Model file for the job. Use its own axes, mm. A direction names the side the tool comes from. Round coordinates to 2 decimals unless told otherwise and drop trailing zeros. Loops run counter-clockwise (first coordinate to the right, second up) from the corner with the lowest first, then second, coordinate; pieces in that order, holes last. Notation, with made-up numbers: (-40, -17) -> (-17, -17) arc R14 cw to (-17, -12) -> close; hole circle Ø7 at (56.5, -34). An arc over 180 degrees is marked (long way). Use a Markdown table: item, result. Add a question column.
```python
from build123d import *

# Parameters (mm, degrees)
SKETCH1_W               = 355.325
SKETCH1_H               = 30
SKETCH1_R               = 12.5
SKETCH1_R_2             = 1
SKETCH1_W_2             = 50
SKETCH1_H_2             = 5
BOSS_EXTRUDE3_DEPTH     = 13
FILLET3_R               = 5
SKETCH3_R               = 12.5
BOSS_EXTRUDE4_DEPTH     = 13
CUT_EXTRUDE1_REACH      = 359.536
SKETCH4_R               = 1.425
SKETCH5_W               = 63.83
SKETCH5_H               = 18
CUT_EXTRUDE3_DEPTH      = 358.535810269
FILLET4_R               = 5
SKETCH6_W               = 63.8325
SKETCH6_H               = 17
CUT_EXTRUDE4_DEPTH      = 5
SKETCH7_R               = 2.159563788
SKETCH7_R_2             = 1
SKETCH7_R_3             = 2.117135705
SKETCH7_R_4             = 1.916104153
SKETCH7_R_5             = 2.415941568
BOSS_EXTRUDE5_DEPTH     = 8
SKETCH8_R               = 12.5
BOSS_EXTRUDE6_DEPTH     = 13
CUT_EXTRUDE5_DEPTH      = 358.535810269
CUT_EXTRUDE5_DEPTH_BACK = 358.535810269
SKETCH10_R              = 12.5
SKETCH10_R_2            = 13
SKETCH13_W              = 13
SKETCH13_H              = 30
BOSS_EXTRUDE7_DEPTH     = 5
SKETCH14_W              = 13
SKETCH14_H              = 9.8
BOSS_EXTRUDE8_DEPTH     = 5
SKETCH15_R              = 1.6
CUT_EXTRUDE6_DEPTH      = 357.119173347
SKETCH17_W              = 5
SKETCH17_H              = 30
CUT_EXTRUDE7_DEPTH      = 357.826085965
BOSS_EXTRUDE9_DEPTH     = 18.5
SKETCH19_W              = 13
SKETCH19_H              = 10.7
BOSS_EXTRUDE10_DEPTH    = 1
CUT_EXTRUDE8_REACH      = 373.267
SKETCH20_W              = 18.5
SKETCH20_H              = 0.75
SKETCH20_W_2            = 18.502042188


with BuildPart() as part:
    # Sketch1 → Boss-Extrude3 (new body)
    # profile 1 of 3: a face of its own
    with BuildSketch(Plane.XY):
        with Locations((177.6625, 15)):
            Rectangle(SKETCH1_W, SKETCH1_H)
        with Locations(Location((334.55, 14.5, 0), (0, 0, 180))):
            Circle(SKETCH1_R, mode=Mode.SUBTRACT)
        with Locations(Location((20.775, 14.5, 0), (0, 0, 180))):
            Circle(SKETCH1_R, mode=Mode.SUBTRACT)
    # profile 2 of 3: a face of its own
    with BuildSketch(Plane.XY):
        Polygon((177.6625, 0), (50, 0), (50, -5), (50, -17), (177.6625, -17), align=None)
        with Locations(Location((60, -14.5, 0), (0, 0, 180))):
            Circle(SKETCH1_R_2, mode=Mode.SUBTRACT)
        with Locations(Location((68, -14.5, 0), (0, 0, 180))):
            Circle(SKETCH1_R_2, mode=Mode.SUBTRACT)
        with Locations(Location((60, -2.5, 0), (0, 0, 180))):
            Circle(SKETCH1_R_2, mode=Mode.SUBTRACT)
        with Locations(Location((68, -2.5, 0), (0, 0, 180))):
            Circle(SKETCH1_R_2, mode=Mode.SUBTRACT)
    # profile 3 of 3: a face of its own
    with BuildSketch(Plane.XY):
        with Locations((25, -2.5)):
            Rectangle(SKETCH1_W_2, SKETCH1_H_2)
    extrude(amount=BOSS_EXTRUDE3_DEPTH)

    # Fillet3
    fillet3_edges = [part.edges().sort_by_distance(p)[0] for p in [
        (0, -5, 6.5),
        (0, 30, 6.5),
        (355.325, 30, 6.5),
        (355.325, 0, 6.5),
        (177.6625, -17, 6.5),
        (50, -17, 6.5),
    ]]
    fillet(fillet3_edges, radius=FILLET3_R)

    # Sketch3 → Boss-Extrude4 (add)
    with BuildSketch(Plane.XY.offset(13)):
        with Locations(Location((85, 14.5, 0), (0, 0, 180))):
            Circle(SKETCH3_R)
        with Locations(Location((165, 14.5, 0), (0, 0, 180))):
            Circle(SKETCH3_R)
        with Locations(Location((245, 14.5, 0), (0, 0, 180))):
            Circle(SKETCH3_R)
    extrude(amount=BOSS_EXTRUDE4_DEPTH)

    # Sketch4 → Cut-Extrude1 (cut, up to next)
    with BuildSketch(Plane(origin=(0, 0, 0), x_dir=(-1, 0, 0), z_dir=(0, 0, -1)), mode=Mode.PRIVATE) as cut_extrude1_sk1:
        with Locations((-68, -2.5)):
            Circle(SKETCH4_R)
    cut_extrude1_tool1 = extrude(cut_extrude1_sk1.sketch, amount=-CUT_EXTRUDE1_REACH, mode=Mode.PRIVATE) & part.part
    # Sketch4 → Cut-Extrude1 (cut, up to next)
    with BuildSketch(Plane(origin=(0, 0, 0), x_dir=(-1, 0, 0), z_dir=(0, 0, -1)), mode=Mode.PRIVATE) as cut_extrude1_sk2:
        with Locations((-60, -2.5)):
            Circle(SKETCH4_R)
    cut_extrude1_tool2 = extrude(cut_extrude1_sk2.sketch, amount=-CUT_EXTRUDE1_REACH, mode=Mode.PRIVATE) & part.part
    # Sketch4 → Cut-Extrude1 (cut, up to next)
    with BuildSketch(Plane(origin=(0, 0, 0), x_dir=(-1, 0, 0), z_dir=(0, 0, -1)), mode=Mode.PRIVATE) as cut_extrude1_sk3:
        with Locations((-60, -14.5)):
            Circle(SKETCH4_R)
    cut_extrude1_tool3 = extrude(cut_extrude1_sk3.sketch, amount=-CUT_EXTRUDE1_REACH, mode=Mode.PRIVATE) & part.part
    # Sketch4 → Cut-Extrude1 (cut, up to next)
    with BuildSketch(Plane(origin=(0, 0, 0), x_dir=(-1, 0, 0), z_dir=(0, 0, -1)), mode=Mode.PRIVATE) as cut_extrude1_sk4:
        with Locations((-68, -14.5)):
            Circle(SKETCH4_R)
    cut_extrude1_tool4 = extrude(cut_extrude1_sk4.sketch, amount=-CUT_EXTRUDE1_REACH, mode=Mode.PRIVATE) & part.part
    add(cut_extrude1_tool1.solids().sort_by_distance((68, -2.5, 0))[0], mode=Mode.SUBTRACT)
    add(cut_extrude1_tool2.solids().sort_by_distance((60, -2.5, 0))[0], mode=Mode.SUBTRACT)
    add(cut_extrude1_tool3.solids().sort_by_distance((60, -14.5, 0))[0], mode=Mode.SUBTRACT)
    add(cut_extrude1_tool4.solids().sort_by_distance((68, -14.5, 0))[0], mode=Mode.SUBTRACT)

    # Sketch5 → Cut-Extrude3 (cut, through all)
    with BuildSketch(Plane(origin=(0, 0, 0), x_dir=(-1, 0, 0), z_dir=(0, 0, -1))):
        with Locations((-145.7475, -9)):
            Rectangle(SKETCH5_W, SKETCH5_H)
    extrude(amount=-CUT_EXTRUDE3_DEPTH, mode=Mode.SUBTRACT)

    # Fillet4
    fillet4_edges = [part.edges().sort_by_distance(p)[0] for p in [
        (113.8325, -17, 6.5),
    ]]
    fillet(fillet4_edges, radius=FILLET4_R)

    # Sketch6 → Cut-Extrude4 (cut)
    with BuildSketch(Plane.XY.offset(13)):
        with Locations((81.91625, -8.5)):
            Rectangle(SKETCH6_W, SKETCH6_H)
    extrude(amount=-CUT_EXTRUDE4_DEPTH, mode=Mode.SUBTRACT)

    # Sketch7 → Boss-Extrude5 (add)
    # profile 1 of 4: a face of its own
    with BuildSketch(Plane.XY.offset(8)):
        with Locations((60, -14.5)):
            Circle(SKETCH7_R)
        with Locations((60, -14.5)):
            Circle(SKETCH7_R_2, mode=Mode.SUBTRACT)
    # profile 2 of 4: a face of its own
    with BuildSketch(Plane.XY.offset(8)):
        with Locations((60, -2.5)):
            Circle(SKETCH7_R_3)
        with Locations((60, -2.5)):
            Circle(SKETCH7_R_2, mode=Mode.SUBTRACT)
    # profile 3 of 4: a face of its own
    with BuildSketch(Plane.XY.offset(8)):
        with Locations((68, -2.5)):
            Circle(SKETCH7_R_4)
        with Locations((68, -2.5)):
            Circle(SKETCH7_R_2, mode=Mode.SUBTRACT)
    # profile 4 of 4: a face of its own
    with BuildSketch(Plane.XY.offset(8)):
        with Locations((68, -14.5)):
            Circle(SKETCH7_R_5)
        with Locations((68, -14.5)):
            Circle(SKETCH7_R_2, mode=Mode.SUBTRACT)
    extrude(amount=-BOSS_EXTRUDE5_DEPTH)

    # Sketch8 → Boss-Extrude6 (add)
    with BuildSketch(Plane.XY.offset(26)):
        with Locations(Location((85, 14.5, 0), (0, 0, 180))):
            Circle(SKETCH8_R)
        with Locations(Location((165, 14.5, 0), (0, 0, 180))):
            Circle(SKETCH8_R)
        with Locations(Location((245, 14.5, 0), (0, 0, 180))):
            Circle(SKETCH8_R)
    extrude(amount=BOSS_EXTRUDE6_DEPTH)

    # Sketch10 → Cut-Extrude5 (cut, two sides: drawn at the far end of the back side and taken through both)
    # profile 1 of 6: a face of its own
    with BuildSketch(Plane.XY.offset(13).offset(-CUT_EXTRUDE5_DEPTH_BACK)):
        with BuildLine():
            Line((285.325, 19.9), (285.325, 30))
            Line((285.325, 30), (5, 30))
            ThreePointArc((5, 30), (1.464466094, 28.535533906), (0, 25))
            Line((0, 25), (0, 0))
            ThreePointArc((0, 0), (1.464466094, -3.535533906), (5, -5))
            Line((5, -5), (50, -5))
            Line((50, -5), (50, 0))
            Line((50, 0), (113.8325, 0))
            Line((113.8325, 0), (285.325, 0))
            Line((285.325, 0), (285.325, 10.1))
            Line((285.325, 10.1), (265.325, 10.1))
            Line((265.325, 10.1), (265.325, 19.9))
            Line((265.325, 19.9), (285.325, 19.9))
        make_face()
        with Locations((20.775, 14.5)):
            Circle(SKETCH10_R, mode=Mode.SUBTRACT)
        with Locations((85, 14.5)):
            Circle(SKETCH10_R, mode=Mode.SUBTRACT)
        with Locations((165, 14.5)):
            Circle(SKETCH10_R, mode=Mode.SUBTRACT)
        with Locations((245, 14.5)):
            Circle(SKETCH10_R, mode=Mode.SUBTRACT)
    # profile 2 of 6: a face of its own
    with BuildSketch(Plane.XY.offset(13).offset(-CUT_EXTRUDE5_DEPTH_BACK)):
        with Locations((334.55, 14.5)):
            Circle(SKETCH10_R_2)
        with Locations((334.55, 14.5)):
            Circle(SKETCH10_R, mode=Mode.SUBTRACT)
    # profile 3 of 6: a face of its own
    with BuildSketch(Plane.XY.offset(13).offset(-CUT_EXTRUDE5_DEPTH_BACK)):
        with Locations((85, 14.5)):
            Circle(SKETCH10_R)
    # profile 4 of 6: a face of its own
    with BuildSketch(Plane.XY.offset(13).offset(-CUT_EXTRUDE5_DEPTH_BACK)):
        with Locations((165, 14.5)):
            Circle(SKETCH10_R)
    # profile 5 of 6: a face of its own
    with BuildSketch(Plane.XY.offset(13).offset(-CUT_EXTRUDE5_DEPTH_BACK)):
        with Locations((245, 14.5)):
            Circle(SKETCH10_R)
    # profile 6 of 6: a face of its own
    with BuildSketch(Plane.XY.offset(13).offset(-CUT_EXTRUDE5_DEPTH_BACK)):
        with BuildLine():
            Line((50, 0), (50, -5))
            Line((50, -5), (50, -12))
            ThreePointArc((50, -12), (51.464466094, -15.535533906), (55, -17))
            Line((55, -17), (108.8325, -17))
            ThreePointArc((108.8325, -17), (112.368033906, -15.535533906), (113.8325, -12))
            Line((113.8325, -12), (113.8325, 0))
            Line((113.8325, 0), (50, 0))
        make_face()
    extrude(amount=CUT_EXTRUDE5_DEPTH + CUT_EXTRUDE5_DEPTH_BACK, mode=Mode.SUBTRACT)

    # Sketch13 → Boss-Extrude7 (add)
    with BuildSketch(Plane.ZY.offset(-285.325)):
        with Locations((6.5, 15)):
            Rectangle(SKETCH13_W, SKETCH13_H)
    extrude(amount=BOSS_EXTRUDE7_DEPTH)

    # Sketch14 → Boss-Extrude8 (add)
    with BuildSketch(Plane.ZY.offset(-265.325)):
        with Locations((6.5, 15)):
            Rectangle(SKETCH14_W, SKETCH14_H)
    extrude(amount=BOSS_EXTRUDE8_DEPTH)

    # Sketch15 → Cut-Extrude6 (cut, through all)
    with BuildSketch(Plane(origin=(0, 19.9, 0), x_dir=(1, 0, 0), z_dir=(0, 1, 0))):
        with Locations(Location((270.325, -6.5, 0), (0, 0, 180))):
            Circle(SKETCH15_R)
    extrude(amount=-CUT_EXTRUDE6_DEPTH, mode=Mode.SUBTRACT)

    # Sketch17 → Cut-Extrude7 (cut, through all)
    with BuildSketch(Plane.XY.offset(13)):
        with Locations((352.825, 15)):
            Rectangle(SKETCH17_W, SKETCH17_H)
    extrude(amount=-CUT_EXTRUDE7_DEPTH, mode=Mode.SUBTRACT)

    # Sketch18 → Boss-Extrude9 (add)
    with BuildSketch(Plane(origin=(350.325, 0, 0), x_dir=(0, 0, -1), z_dir=(1, 0, 0))):
        Polygon((-11.25, 30), (-11.25, 1.5), (-1.75, 1.5), (-1.75, 30), (0, 30), (0, 0), (-13, 0), (-13, 30), align=None)
    extrude(amount=BOSS_EXTRUDE9_DEPTH)

    # Sketch19 → Boss-Extrude10 (add)
    with BuildSketch(Plane(origin=(368.825, 0, 0), x_dir=(0, 0, -1), z_dir=(1, 0, 0))):
        with Locations((-6.5, 24.65)):
            Rectangle(SKETCH19_W, SKETCH19_H)
    extrude(amount=BOSS_EXTRUDE10_DEPTH)

    # Cut-Extrude8: up to this face of the body (flat: up to its plane)
    cut_extrude8_end = Plane(part.part.faces().sort_by_distance((359.575, 1.5, 6.5))[0])
    # Sketch20 → Cut-Extrude8 (cut, up to the picked face)
    with BuildSketch(Plane(origin=(0, 30, 0), x_dir=(1, 0, 0), z_dir=(0, 1, 0)), mode=Mode.PRIVATE) as cut_extrude8_sk1:
        with Locations((359.575, -1.375)):
            Rectangle(SKETCH20_W, SKETCH20_H)
    cut_extrude8_tool1 = split(extrude(cut_extrude8_sk1.sketch, amount=-CUT_EXTRUDE8_REACH, mode=Mode.PRIVATE), bisect_by=cut_extrude8_end, keep=Keep.BOTH, mode=Mode.PRIVATE)
    # Sketch20 → Cut-Extrude8 (cut, up to the picked face)
    with BuildSketch(Plane(origin=(0, 30, 0), x_dir=(1, 0, 0), z_dir=(0, 1, 0)), mode=Mode.PRIVATE) as cut_extrude8_sk2:
        with Locations((359.576021094, -11.625)):
            Rectangle(SKETCH20_W_2, SKETCH20_H)
    cut_extrude8_tool2 = split(extrude(cut_extrude8_sk2.sketch, amount=-CUT_EXTRUDE8_REACH, mode=Mode.PRIVATE), bisect_by=cut_extrude8_end, keep=Keep.BOTH, mode=Mode.PRIVATE)
    add(cut_extrude8_tool1.solids().sort_by(Axis((359.575, 30, 1.375), (0, -1, 0)))[0], mode=Mode.SUBTRACT)
    add(cut_extrude8_tool2.solids().sort_by(Axis((359.576021, 30, 11.625), (0, -1, 0)))[0], mode=Mode.SUBTRACT)


solid = part.part
```
1) Pin check, flat tips, straight feed: pin 1 Ø0.5 at (x, z) = (369.5, 6) entering from -Y; pin 2 Ø4 at (x, z) = (271, 8) entering from +Y; pin 3 Ø5 at (y, z) = (24, 6) entering from -X (3 decimals). Stop position of each tip, or through.
2) Cut at B-B on y = 14.5. Write the cut outline in (x, z) (3 decimals).
3) Pull direction Z, two halves, no side cores. Call faces 4 (the face through (314, 15, 13)), 5 (the face through (369.825, 25, 7)), 6 (the face through (359, 16, 1)): +Z half, -Z half, draft (parallel to the pull), parting line (faces both ways), or undercut.
4) Cut at C-C on x = 334.55. Write the cut outline in (y, z), and give its area (3 significant figures).
5) Cut at A-A on z = 6.5. Write the cut outline in (x, y) (3 decimals), and give its area (3 significant figures).
6) Wall check: probe 1 along Z at (x, y) = (354.5, 19); probe 2 along X at (y, z) = (14.5, 9.25) (3 decimals); probe 3 along Y at (x, z) = (334.55, 6). Give the ranges that are in metal, low to high. Write a range as from..to.
7) Tool access for faces 1 (the face through (280.325, 25, 6)), 2 (the face through (359, 1.5, 7)), 3 (the face through (359, 16, 12)): list every direction of +Z, -Z, +X, -X, +Y, -Y with a clear straight run to the whole face (end or side of a thin tool).
8) Cut at D-D on x = 351.5. Write the cut outline in (y, z).
Established:
| question | item | result |
|---|---|---|
| 1 | pin 1 | stops at y = 19.3 |
| 1 | pin 2 | stops at y = 19.9 |
| 1 | pin 3 | stops at x = 280.325 |
| 2 | outline | (260.325, 0) -> (321.55, 0) -> (321.55, 13) -> (260.325, 13) -> close; (347.55, 0) -> (368.825, 0) -> (368.825, 1) -> (350.325, 1) -> (350.325, 12) -> (368.825, 12) -> (368.825, 13) -> (347.55, 13) -> close; hole circle Ø3.2 at (270.325, 6.5) |
| 3 | face 4 | +Z half |
| 3 | face 5 | draft |
| 3 | face 6 | undercut |
| 4 | outline | (0, 0) -> (1.5, 0) -> (1.5, 13) -> (0, 13) -> close; (27.5, 0) -> (30, 0) -> (30, 13) -> (27.5, 13) -> close |
| 4 | area | 52.0 mm^2 |
| 5 | outline | (260.325, 10.1) -> (268.725, 10.1) -> (268.725, 19.9) -> (260.325, 19.9) -> close; (271.925, 10.1) -> (280.325, 10.1) -> (280.325, 0) -> (368.825, 0) -> (368.825, 1.5) -> (350.325, 1.5) -> (350.325, 30) -> (280.325, 30) -> (280.325, 19.9) -> (271.925, 19.9) -> close; (368.825, 19.3) -> (369.825, 19.3) -> (369.825, 30) -> (368.825, 30) -> close; hole circle Ø26 at (334.55, 14.5) |
| 5 | area | 1,770 mm^2 |
| 6 | probe 1 | z = 0..1, 12..13 |
| 6 | probe 2 | x = 260.325..321.55, 347.55..350.325 |
| 6 | probe 3 | y = 0..1.5, 27.5..30 |
| 7 | face 1 | +Z, -Z, -X, +Y |
| 7 | face 2 | +X, +Y |
| 7 | face 3 | +Y |
| 8 | outline | (0, 0) -> (30, 0) -> (30, 1) -> (1.5, 1) -> (1.5, 12) -> (30, 12) -> (30, 13) -> (0, 13) -> close |
